```python
from build123d import *

# Parameters (mm, degrees)
SKETCH_1_W          = 15
SKETCH_1_H          = 20
EXTRUDE_1_DEPTH     = 55
SKETCH_3_W          = 2
SKETCH_3_H          = 6
EXTRUDE_2_DEPTH     = 1
SKETCH_4_W          = 2
SKETCH_4_H          = 2
EXTRUDE_3_DEPTH     = 2
SKETCH_5_W          = 6.633447251
SKETCH_5_H          = 20.27238771
SKETCH_5_W_2        = 12.16711561
SKETCH_5_H_2        = 23.052373823
CUT_EXTRUDE_1_DEPTH = 24
SKETCH_6_R          = 1
EXTRUDE_4_DEPTH     = 10


with BuildPart() as part:
    # 草图1 → 凸台-拉伸1 (new body)
    with BuildSketch(Plane(origin=(0, 0, 0), x_dir=(0, 0, -1), z_dir=(1, 0, 0))):
        Rectangle(SKETCH_1_W, SKETCH_1_H)
    extrude(amount=EXTRUDE_1_DEPTH)

    # 草图2 → 旋转1 (revolve)
    with BuildSketch(Plane.XY):
        with BuildLine():
            Line((55, 0), (70, 0))
            Line((70, 0), (70, 7.947586675))
            ThreePointArc((70, 7.947586675), (69.417060699, 9.358947358), (68.008061024, 9.94757043))
            Line((68.008061024, 9.94757043), (55, 10))
            Line((55, 10), (55, 0))
        make_face()
    revolve(axis=Axis((55, 0, 0), (1, 0, 0)))

    # 草图3 → 凸台-拉伸2 (add)
    with BuildSketch(Plane(origin=(0, 0, -7.5), x_dir=(-1, 0, 0), z_dir=(0, 0, -1))):
        with Locations((-54, 7)):
            Rectangle(SKETCH_3_W, SKETCH_3_H)
        with Locations((-54, -7)):
            Rectangle(SKETCH_3_W, SKETCH_3_H)
    extrude(amount=EXTRUDE_2_DEPTH)

    # 草图4 → 凸台-拉伸3 (add)
    with BuildSketch(Plane.XY.offset(7.5)):
        with Locations((20, 0)):
            Rectangle(SKETCH_4_W, SKETCH_4_H)
    extrude(amount=EXTRUDE_3_DEPTH)

    # 草图5 → 切除-拉伸1 (cut)
    with BuildSketch(Plane.ZY.offset(-55)):
        with Locations((-10.816723626, -0.136193855)):
            Rectangle(SKETCH_5_W, SKETCH_5_H)
        with Locations((13.583557805, -1.526186911)):
            Rectangle(SKETCH_5_W_2, SKETCH_5_H_2)
    extrude(amount=-CUT_EXTRUDE_1_DEPTH, mode=Mode.SUBTRACT)

    # 草图6 → 凸台-拉伸4 (add)
    with BuildSketch(Plane.XY.offset(9.5)):
        with Locations((20, 0)):
            Circle(SKETCH_6_R)
    extrude(amount=EXTRUDE_4_DEPTH)


solid = part.part
```
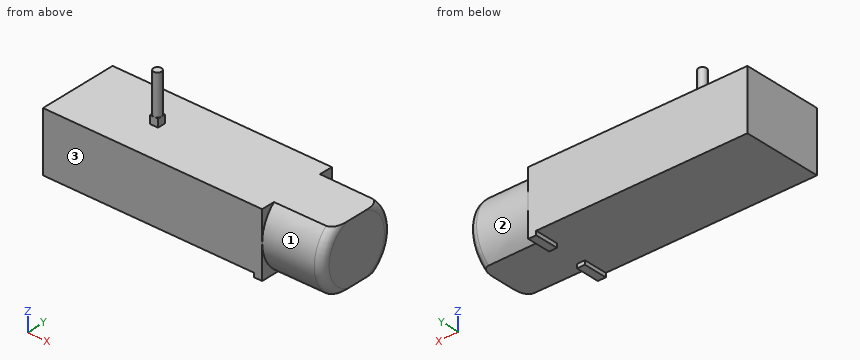
Verification items for the finished model (mm, model axes). Face numbers are marked on the shaded views. A direction names the side the tool comes from. Round coordinates to 2 decimals unless told otherwise and drop trailing zeros. Write each loop counter-clockwise with the first axis right and the second up, starting at its lowest first coordinate (ties: lowest second). Pieces come first, ordered by that corner, then holes. Notation, with made-up numbers: (-26.5, 66.5) - (8.5, 66.5) arc R21 ccw to (8.5, 81.5) - close; hole circle Ø10 at (86, -34.5). An arc over 180 degrees is marked (long way). Answer as a JSON object with one key per item and string values. Group by question number.
Q1. Go/stop test with flat-tipped pins: pin 1 Ø1 at (y, z) = (-0.5, 8.5) entering from -X; pin 2 Ø10 at (x, y) = (19, 2) entering from -Z; pin 3 Ø6 at (x, y) = (25, 0.5) entering from +Z. Record where each tip stops, or that it passes through.
Q2. Section check C-C, the plane x = 62.5. Enter the section's corners in (y, z), plus the area to 3 significant figures.
Q3. Thickness scan on line 1 (Z direction, x = 28.5, y = 7.25); line 2 (Z direction, x = 65, y = -7.5); line 3 (X direction, y = -9, z = -6.5). Record the ranges inside material, lowest first.
Q4. Section check A-A, the plane x = 52. Enter the section's corners in (y, z).
Q5. Tool access check on the marked faces 1, 2 and 3. Record the directions out of +Z, -Z, +X, -X, +Y, -Y that give a thin tool (end or side, any length) a straight path to the whole face; none if there is none.
Q6. Section check B-B, the plane z = 17.25. Enter the section's corners in (x, y).
Found:
{
 "1": {"pin 1": "stops at x = 19", "pin 2": "stops at z = -7.5", "pin 3": "stops at z = 7.5"},
 "2": {"outline": "(-6.57, -7.5) - (6.57, -7.5) arc R9.97 ccw to (6.57, 7.5) - (-6.57, 7.5) arc R9.97 ccw to start", "area": "268 mm^2"},
 "3": {"line 1": "z = -7.5 to 7.5", "line 2": "z = -6.55 to 6.55", "line 3": "x = 0 to 55"},
 "4": {"outline": "(-10, -7.5) - (10, -7.5) - (10, 7.5) - (-10, 7.5) - close"},
 "5": {"face 1": "+X, -Y", "face 2": "+X, +Y", "face 3": "+Z, -Z, +X, -X, -Y"},
 "6": {"outline": "circle Ø2 at (20, 0)"}
}
